The drawing under review shows one solid part. Ordinate dimensions are in mm from its lowest x, y, z. A direction names the side the tool comes from. Give positions to 0.01 mm unless a question says otherwise; leave off trailing zeros. Loops run counter-clockwise (first coordinate to the right, second up) from the corner with the lowest first, then second, coordinate; pieces in that order, holes last. Notation, with made-up numbers: (-32, 86.25) - (-1, 86.25) arc R21 cw to (-1, 98.25) - close; hole circle Ø2 at (85.5, 7). An arc over 180 degrees is marked (long way). Answer as CSV lines item,"result".
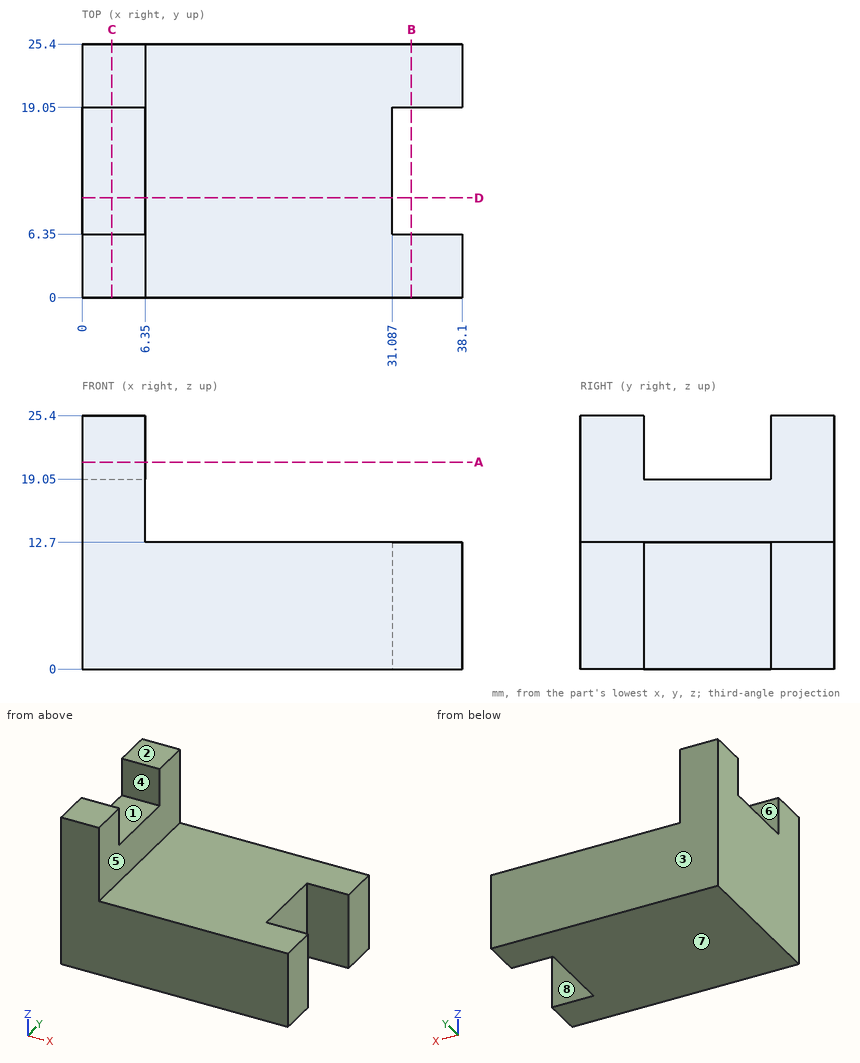
1) Draft analysis for pull direction Y (two halves, no side actions). For the marked faces 1, 2, 3 and 4, state which applies: pulls with the +Y half, pulls with the -Y half, needs draft (parallel to the pull), parting line crosses it, or undercut.
From the geometry:
face 1,"undercut"
face 2,"needs draft"
face 3,"pulls with the +Y half"
face 4,"undercut"
2) Machinability: for the marked faces 5, 6, 7 and 8, which of the approach directions +Z, -Z, +X, -X, +Y, -Y give a long, thin tool a straight path to every point of the face, cutting with its end or side? Answer none if there is none.
From the geometry:
face 5,"+Z, +X, +Y, -Y"
face 6,"+Z, +X, -X"
face 7,"-Z, +X, -X, +Y, -Y"
face 8,"+Z, -Z, +X"
3) Consider section A-A on z = 20.75. Write out the cut boundary in (x, y).
From the geometry:
outline,"(0, 0) - (6.35, 0) - (6.35, 6.35) - (0, 6.35) - close; (0, 19.05) - (6.35, 19.05) - (6.35, 25.4) - (0, 25.4) - close"
4) Consider section C-C on x = 3. Write out the cut boundary in (y, z), and give its area (4 significant figures).
From the geometry:
outline,"(0, 0) - (25.4, 0) - (25.4, 25.4) - (19.05, 25.4) - (19.05, 19.05) - (6.35, 19.05) - (6.35, 25.4) - (0, 25.4) - close"
area,"564.5 mm^2"
5) Wall thickness on line 1 (Z direction, x = 34, y = 6); line 2 (X direction, y = 3.5, z = 14); line 3 (X direction, y = 8.5, z = 10.25): over which ranges is each line inside the solid? List them lowest first. Write a range as from..to.
From the geometry:
line 1,"z = 0..12.7"
line 2,"x = 0..6.35"
line 3,"x = 0..31.09"
6) Consider section D-D on y = 10. Write out the cut boundary in (x, z).
From the geometry:
outline,"(0, 0) - (31.09, 0) - (31.09, 12.7) - (6.35, 12.7) - (6.35, 19.05) - (0, 19.05) - close"
7) Insertion check: P1, Ø4, axis at y = 16, z = 17.5, coming from the +X side; P2, Ø4, axis at x = 9.5, y = 5, coming from the +Z side; P3, Ø5, axis at x = 1.5, y = 14, coming from the +Z side. Each pin has a flat end and moves straight along its axis. Give the tip position at first contact, or say it passes through.
From the geometry:
P1,"stops at x = 6.35"
P2,"stops at z = 12.7"
P3,"stops at z = 19.05"
8) Consider section B-B on x = 33. Write out the cut boundary in (y, z), and give its area (3 significant figures).
From the geometry:
outline,"(0, 0) - (6.35, 0) - (6.35, 12.7) - (0, 12.7) - close; (19.05, 0) - (25.4, 0) - (25.4, 12.7) - (19.05, 12.7) - close"
area,"161 mm^2"
